Input: dimensioned drawing with shaded views. Units: mm. Origin: part minimum x, y, z. Coordinates: 2 decimals unless noted, no trailing zeros. Write each loop counter-clockwise with the first axis right and the second up, starting at its lowest first coordinate (ties: lowest second). Pieces come first, ordered by that corner, then holes. Notation, with made-up numbers: (-40, -33.5) -> (-14, -33.5) arc R17 ccw to (-14, -27.5) -> close; hole circle Ø4 at (-14, 53.25). An arc over 180 degrees is marked (long way). One line per item, written item: value. Start each with the question number.
1. Section query B-B, the plane x = 9. Output: boundary loops of the cut face in (y, z) (1 decimal).
2. Section query C-C, the plane y = 1.95. Output: boundary loops of the cut face in (x, z) (1 decimal), and give its area (3 significant figures).
3. Section query A-A, the plane z = 24. Output: boundary loops of the cut face in (x, y) (1 decimal).
4. Line query: line 1 (X direction, y = 0.8, z = 25.5) (1 decimal); line 2 (Z direction, x = 15.5, y = 0.95) (1 decimal); line 3 (Z direction, x = 12.25, y = 3.3) (1 decimal). Output: solid intervals per line, ascending.
5. First-contact query: P1, Ø0.8, axis at y = 2.5, z = 1.5, coming from the +X side; P2, Ø6.5, axis at x = 11.5, z = 24.5, coming from the +Y side. Flat tips, straight axial feed; report the tip coordinate or a pass-through.
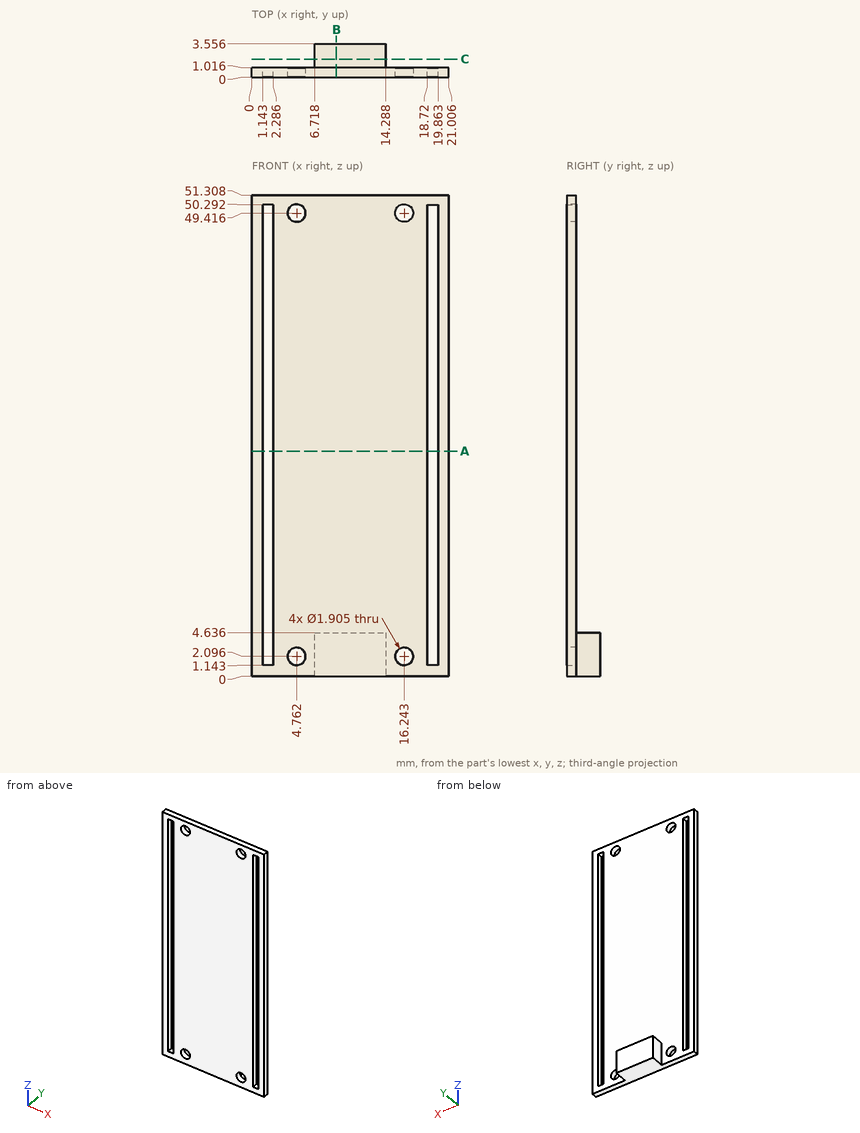
Computed values:
1. outline: (0, 0) -> (3.6, 0) -> (3.6, 4.6) -> (1, 4.6) -> (1, 51.3) -> (0, 51.3) -> close
2. outline: (6.7, 0) -> (14.3, 0) -> (14.3, 4.6) -> (6.7, 4.6) -> close
2. area: 35.1 mm²
3. outline: (0, 0) -> (1.1, 0) -> (1.1, 1) -> (0, 1) -> close; (2.3, 0) -> (18.7, 0) -> (18.7, 1) -> (2.3, 1) -> close; (19.9, 0) -> (21, 0) -> (21, 1) -> (19.9, 1) -> close
4. line 1: x = 0 to 1.1, 2.3 to 18.7, 19.9 to 21
4. line 2: z = 0 to 1.5, 2.7 to 48.8, 50 to 51.3
4. line 3: z = 0 to 4.6
5. P1: stops at x = 14.29
5. P2: stops at y = 1.02
